Geometry check sheet. Reference: the model listing, model coordinates, mm. Face numbers are marked on the shaded views. A direction names the side the tool comes from. Coordinates: 2 decimals unless noted, no trailing zeros. Loops run counter-clockwise (first coordinate to the right, second up) from the corner with the lowest first, then second, coordinate; pieces in that order, holes last. Notation, with made-up numbers: (83, -16.5) - (118, -16.5) arc R25 ccw to (118, 12.5) - close; hole circle Ø9 at (65.5, 11). An arc over 180 degrees is marked (long way). One line per item, written item: value.
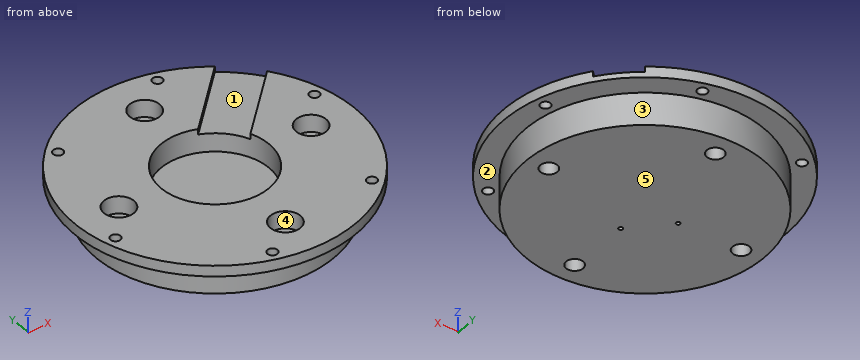
from build123d import *

# Parameters (mm, degrees)
F0_R      = 41.275
F1_DEPTH  = 3.175
F2_R      = 34.925
F3_DEPTH  = 9.525
F4_R      = 2.4892
F5_DEPTH  = 12.7
F6_R      = 4.4196
F7_DEPTH  = 5.08
F8_R      = 1.4732
F9_DEPTH  = 3.175
F10_R     = 15.875
F11_DEPTH = 6.985
F12_R     = 0.59563
F13_DEPTH = 5.716
F15_DEPTH = 1.5875


with BuildPart() as f1:
    # F0 (on Top) → F1 (new body)
    with BuildSketch(Plane.XY):
        Circle(F0_R)
    extrude(amount=F1_DEPTH)

    # F2 (on face) → F3 (join)
    with BuildSketch(Plane(origin=(0, 0, 0), x_dir=(1, 0, 0), z_dir=(0, 0, -1))):
        Circle(F2_R)
    extrude(amount=F3_DEPTH)

    # F4 (on face) → F5 (cut, through all)
    with BuildSketch(Plane.XY.offset(3.175)):
        with Locations((0, 28.575)):
            Circle(F4_R)
        with Locations((-28.575, 0)):
            Circle(F4_R)
        with Locations((0, -28.575)):
            Circle(F4_R)
        with Locations((28.575, 0)):
            Circle(F4_R)
    extrude(amount=-F5_DEPTH, mode=Mode.SUBTRACT)

    # F6 (on face) → F7 (cut)
    with BuildSketch(Plane.XY.offset(3.175)):
        with Locations((0, 28.575)):
            Circle(F6_R)
        with Locations((-28.575, 0)):
            Circle(F6_R)
        with Locations((0, -28.575)):
            Circle(F6_R)
        with Locations((28.575, 0)):
            Circle(F6_R)
    extrude(amount=-F7_DEPTH, mode=Mode.SUBTRACT)

    # F8 (on face) → F9 (cut, through all)
    with BuildSketch(Plane(origin=(0, 0, 0), x_dir=(1, 0, 0), z_dir=(0, 0, -1))):
        with Locations((9.8610056184, -36.8017739816)):
            Circle(F8_R)
        with Locations((36.8017739816, -9.8610056184)):
            Circle(F8_R)
        with Locations((26.9407683632, 26.9407683632)):
            Circle(F8_R)
        with Locations((-9.8610056184, 36.8017739816)):
            Circle(F8_R)
        with Locations((-36.8017739816, 9.8610056184)):
            Circle(F8_R)
        with Locations((-26.9407683632, -26.9407683632)):
            Circle(F8_R)
    extrude(amount=-F9_DEPTH, mode=Mode.SUBTRACT)

    # F10 (on face) → F11 (cut)
    with BuildSketch(Plane.XY.offset(3.175)):
        Circle(F10_R)
    extrude(amount=-F11_DEPTH, mode=Mode.SUBTRACT)

    # F12 (on face) → F13 (cut, through all)
    with BuildSketch(Plane.XY.offset(-3.81)):
        with Locations((-9.8782817332, 0)):
            Circle(F12_R)
        with Locations((0, -9.8782817332)):
            Circle(F12_R)
    extrude(amount=-F13_DEPTH, mode=Mode.SUBTRACT)

    # F14 (on face) → F15 (cut)
    with BuildSketch(Plane.XY.offset(3.175)):
        with BuildLine():
            Line((24.3482415622, 33.3284976833), (5.7980477982, 14.7783039193))
            ThreePointArc((5.7980477982, 14.7783039193), (11.2253201513, 11.2253201513), (14.7783039193, 5.7980477982))
            Line((14.7783039193, 5.7980477982), (33.3284976833, 24.3482415622))
            ThreePointArc((33.3284976833, 24.3482415622), (29.1858323935, 29.1858323935), (24.3482415622, 33.3284976833))
        make_face()
    extrude(amount=-F15_DEPTH, mode=Mode.SUBTRACT)


solid = f1.part
(1) Cross-section at D-D on y = -12.5. Record the cut outline in (x, z) (3 decimals).
Reply:
outline: (-39.337, 0) - (-32.611, 0) - (-32.611, -9.525) - (32.611, -9.525) - (32.611, 0) - (39.337, 0) - (39.337, 3.175) - (9.786, 3.175) - (9.786, -3.81) - (-9.786, -3.81) - (-9.786, 3.175) - (-39.337, 3.175) - close
(2) Go/stop test with flat-tipped pins: pin 1 Ø7 at (x, y) = (-28.575, 0) entering from +Z (3 decimals); pin 2 Ø9.5 at (x, y) = (0, -4) entering from +Z; pin 3 Ø3 at (x, z) = (20.5, -2.5) entering from +Y. Record where each tip stops, or that it passes through.
Reply:
pin 1: z = -1.905
pin 2: z = -3.81
pin 3: y = 29.3
(3) Cross-section at A-A on x = 29.5. Record the cut outline in (y, z) (1 decimal).
Reply:
outline: (-28.9, 0) - (-18.7, 0) - (-18.7, -9.5) - (-2.3, -9.5) - (-2.3, -1.9) - (-4.3, -1.9) - (-4.3, 3.2) - (-28.9, 3.2) - close; (2.3, -9.5) - (18.7, -9.5) - (18.7, 0) - (28.9, 0) - (28.9, 1.6) - (20.5, 1.6) - (20.5, 3.2) - (4.3, 3.2) - (4.3, -1.9) - (2.3, -1.9) - close
(4) Access from +Z, -Z, +X, -X, +Y, -Y to the whole of each face (thin tool, end or side, straight path). Record for the marked faces 4 and 5.
Reply:
face 4: +Z
face 5: -Z, +X, -X, +Y, -Y
(5) Material ranges on probe 1 along Y at (x, z) = (0, -6.25) (3 decimals); probe 2 along X at (y, z) = (1.5, -4.5); probe 3 along X at (y, z) = (-2.5, 2.5), recorded low to high. Write a range as from..to.
Reply:
probe 1: -34.925..-31.064, -26.086..-10.474, -9.283..26.086, 31.064..34.925
probe 2: -34.89..-30.56, -26.59..26.59, 30.56..34.89
probe 3: -41.2..-32.22, -24.93..-15.68, 15.68..24.93, 32.22..41.2
(6) Cross-section at C-C on y = 22. Record the cut outline in (x, z) (1 decimal).
Reply:
outline: (-34.9, 0) - (-27.1, 0) - (-27.1, -9.5) - (27.1, -9.5) - (27.1, 0) - (34.9, 0) - (34.9, 3.2) - (31, 3.2) - (31, 1.6) - (13, 1.6) - (13, 3.2) - (-34.9, 3.2) - close
(7) Release check for a two-part mould opening along Y. For the marked faces 1, 2 and 3 record: pulls with the +Y half, pulls with the -Y half, needs draft (parallel to the pull), parting line crosses it, or undercut.
Reply:
face 1: undercut
face 2: needs draft
face 3: parting line crosses it
(8) Cross-section at B-B on z = -6. Record the cut outline in (x, y) (3 decimals).
Reply:
outline: circle Ø69.85 at (0, 0); hole circle Ø4.978 at (-28.575, 0); hole circle Ø1.191 at (-9.878, 0); hole circle Ø4.978 at (0, -28.575); hole circle Ø4.978 at (0, 28.575); hole circle Ø1.191 at (0, -9.878); hole circle Ø4.978 at (28.575, 0)
